Build history of the part. All positions in model axes, mm. Face numbers are marked on the shaded views. A direction names the side the tool comes from. Round coordinates to 2 decimals unless told otherwise and drop trailing zeros. Write each loop counter-clockwise with the first axis right and the second up, starting at its lowest first coordinate (ties: lowest second). Pieces come first, ordered by that corner, then holes. Notation, with made-up numbers: (49, 36) - (60, 36) arc R19 cw to (60, 46) - close; hole circle Ø6 at (37.5, 50). An arc over 180 degrees is marked (long way). Write each question's results on one line, items separated by ' | '.
from build123d import *

# Parameters (mm, degrees)
SKETCH1_W           = 32
SKETCH1_H           = 12
BOSS_EXTRUDE1_DEPTH = 2
SKETCH2_W           = 22
SKETCH2_H           = 12
BOSS_EXTRUDE2_DEPTH = 15
SKETCH3_W           = 22
SKETCH3_H           = 12
BOSS_EXTRUDE3_DEPTH = 4
BOSS_EXTRUDE4_DEPTH = 4
BOSS_EXTRUDE5_DEPTH = 4
SKETCH6_R           = 2.5
SKETCH6_R_2         = 0.75
BOSS_EXTRUDE6_DEPTH = 2
SKETCH7_R           = 1
SKETCH7_W           = 5
SKETCH7_H           = 1
CUT_EXTRUDE1_DEPTH  = 25.103941586
FILLET1_R           = 0.3
SKETCH8_W           = 1.18990991
SKETCH8_H           = 0.976336336
SKETCH8_H_2         = 0.976336337
BOSS_EXTRUDE7_DEPTH = 0.1


with BuildPart() as part:
    # Sketch1 → Boss-Extrude1 (new body)
    with BuildSketch(Plane(origin=(0, 0, 0), x_dir=(1, 0, 0), z_dir=(0, 1, 0))):
        Rectangle(SKETCH1_W, SKETCH1_H)
    extrude(amount=BOSS_EXTRUDE1_DEPTH)

    # Sketch2 → Boss-Extrude2 (add)
    with BuildSketch(Plane.XZ):
        Rectangle(SKETCH2_W, SKETCH2_H)
    extrude(amount=BOSS_EXTRUDE2_DEPTH)

    # Sketch3 → Boss-Extrude3 (add)
    with BuildSketch(Plane(origin=(0, 2, 0), x_dir=(1, 0, 0), z_dir=(0, 1, 0))):
        Rectangle(SKETCH3_W, SKETCH3_H)
    extrude(amount=BOSS_EXTRUDE3_DEPTH)

    # Sketch4 → Boss-Extrude4 (add)
    with BuildSketch(Plane(origin=(0, 6, 0), x_dir=(1, 0, 0), z_dir=(0, 1, 0))):
        with BuildLine():
            ThreePointArc((9.242640687, 4.242640687), (7.296100594, 5.543277195), (5, 6))
            ThreePointArc((5, 6), (0.757359313, 4.242640687), (-1, 0))
            ThreePointArc((-1, 0), (-0.543277195, -2.296100594), (0.757359313, -4.242640687))
            Line((0.757359313, -4.242640687), (9.242640687, 4.242640687))
        make_face()
        with BuildLine():
            ThreePointArc((11, 0), (10.543277195, 2.296100594), (9.242640687, 4.242640687))
            Line((9.242640687, 4.242640687), (0.757359313, -4.242640687))
            ThreePointArc((0.757359313, -4.242640687), (7.296100594, -5.543277195), (11, 0))
        make_face()
    extrude(amount=BOSS_EXTRUDE4_DEPTH)

    # Sketch5 → Boss-Extrude5 (add)
    with BuildSketch(Plane(origin=(0, 6, 0), x_dir=(1, 0, 0), z_dir=(0, 1, 0))):
        with BuildLine():
            ThreePointArc((-1, 0), (-0.862002062, 1.279426367), (-0.454356057, 2.5))
            Line((-0.454356057, 2.5), (-2, 2.5))
            ThreePointArc((-2, 2.5), (-4.5, 0), (-2, -2.5))
            Line((-2, -2.5), (-0.454356057, -2.5))
            ThreePointArc((-0.454356057, -2.5), (-0.862002062, -1.279426367), (-1, 0))
        make_face()
    extrude(amount=BOSS_EXTRUDE5_DEPTH)

    # Sketch6 → Boss-Extrude6 (add)
    with BuildSketch(Plane(origin=(0, 10, 0), x_dir=(1, 0, 0), z_dir=(0, 1, 0))):
        with Locations(Location((5, 0, 0), (0, 0, 270))):
            Circle(SKETCH6_R)
        with Locations(Location((5, 0, 0), (0, 0, 270))):
            Circle(SKETCH6_R_2, mode=Mode.SUBTRACT)
    extrude(amount=BOSS_EXTRUDE6_DEPTH)

    # Sketch7 → Cut-Extrude1 (cut, through all)
    with BuildSketch(Plane(origin=(0, 2, 0), x_dir=(1, 0, 0), z_dir=(0, 1, 0))):
        with Locations((14, 0)):
            Circle(SKETCH7_R)
        with Locations((-14, 0)):
            Circle(SKETCH7_R)
        with Locations((16, 0)):
            Rectangle(SKETCH7_W, SKETCH7_H)
        with Locations((-16, 0)):
            Rectangle(SKETCH7_W, SKETCH7_H)
    extrude(amount=-CUT_EXTRUDE1_DEPTH, mode=Mode.SUBTRACT)

    # Fillet1
    fillet1_edges = [part.edges().sort_by_distance(p)[0] for p in [
        (11, 4, -6),
        (11, -7.5, -6),
        (11, 4, 6),
        (11, -7.5, 6),
        (-11, 4, -6),
        (-11, 4, 6),
        (-11, -7.5, 6),
        (-11, -7.5, -6),
        (-16, 1, -6),
        (-16, 1, 6),
        (16, 1, -6),
        (16, 1, 6),
    ]]
    fillet(fillet1_edges, radius=FILLET1_R)

    # Sketch8 → Boss-Extrude7 (add)
    # profile 1 of 10: a face of its own
    with BuildSketch(Plane.XY.offset(6)):
        Polygon((-6.546228955, -2.789688189), (-7.217460186, -2.789688189), (-7.217460186, -1.581662663), (-7.868192168, -2.564673174), (-8.295339315, -2.564673174), (-8.926048774, -1.582616117), (-8.926048774, -2.775386387), (-9.597280006, -3.125303805), (-9.597280006, -0.837015516), (-8.876469195, -0.837015516), (-8.079858834, -1.98115966), (-7.268469946, -0.837015516), (-6.546228955, -0.837015516), align=None)
    # profile 2 of 10: a face of its own
    with BuildSketch(Plane.XY.offset(6)):
        Polygon((-5.569892618, -2.778246748), (-6.241123849, -3.125303805), (-6.241123849, -0.837015516), (-5.569892618, -0.837015516), align=None)
    # profile 3 of 10: a face of its own
    with BuildSketch(Plane.XY.offset(6)):
        Polygon((-2.923582558, -0.837015516), (-3.373135861, -1.325183685), (-4.624066792, -1.325183685), (-4.624066792, -2.301520021), (-2.99175448, -2.301520021), (-3.445121597, -2.789688189), (-4.84431454, -2.789688189), (-5.295298024, -2.344902153), (-5.295298024, -1.285138639), (-4.84431454, -0.837015516), align=None)
    # profile 4 of 10: a face of its own
    with BuildSketch(Plane.XY.offset(6)):
        Polygon((-0.2915743, -2.789688189), (-0.962805531, -2.789688189), (-0.962805531, -2.31772873), (-1.138717693, -2.148967468), (-2.152715441, -2.148967468), (-2.152715441, -2.770142393), (-2.823946672, -3.125303805), (-2.823946672, -0.837015516), (-0.762580306, -0.837015516), (-0.2915743, -1.45103954), (-0.63672445, -1.892488489), (-0.2915743, -2.219999751), align=None)
        Polygon((-0.981397873, -1.52397873), (-1.143008234, -1.325183685), (-2.152715441, -1.325183685), (-2.152715441, -1.6607993), (-1.096765741, -1.6607993), align=None, mode=Mode.SUBTRACT)
    # profile 5 of 10: a face of its own
    with BuildSketch(Plane.XY.offset(6)):
        Polygon((2.545903178, -2.332507258), (2.08824552, -2.789688189), (0.461653928, -2.789688189), (0.013530805, -2.342041793), (0.013530805, -1.285138639), (0.462130655, -0.837015516), (2.087768793, -0.837015516), (2.545903178, -1.294673174), align=None)
        with Locations((1.279716991, -1.813351853)):
            Rectangle(SKETCH8_W, SKETCH8_H, mode=Mode.SUBTRACT)
    # profile 6 of 10: a face of its own
    with BuildSketch(Plane.XY.offset(6)):
        Polygon((-1.064397577, -5.019272635), (-1.519194874, -5.623285398), (-3.801285715, -5.623285398), (-3.361266946, -5.13511723), (-1.916784964, -5.13511723), (-1.799033463, -5.025946809), (-1.91154097, -4.891033146), (-3.366987667, -4.891033146), (-3.801285715, -4.292741103), (-3.352685865, -3.670612725), (-1.064397577, -3.670612725), (-1.517764694, -4.158780893), (-2.964153583, -4.158780893), (-3.079044724, -4.29178765), (-2.963200129, -4.433375488), (-1.507753433, -4.433375488), align=None)
    # profile 7 of 10: a face of its own
    with BuildSketch(Plane.XY.offset(6)):
        Polygon((1.52994927, -3.670612725), (1.080395967, -4.158780893), (-0.170534964, -4.158780893), (-0.170534964, -4.433375488), (1.251540862, -4.433375488), (0.837265336, -4.891033146), (-0.170534964, -4.891033146), (-0.170534964, -5.13511723), (1.461777348, -5.13511723), (1.008410231, -5.623285398), (-0.841766195, -5.623285398), (-0.841766195, -3.670612725), align=None)
    # profile 8 of 10: a face of its own
    with BuildSketch(Plane.XY.offset(6)):
        Polygon((4.222978549, -5.623285398), (3.551747318, -5.623285398), (3.551747318, -5.151325938), (3.375835156, -4.982564677), (2.361837408, -4.982564677), (2.361837408, -5.603739602), (1.690606177, -5.958901013), (1.690606177, -3.670612725), (3.751972543, -3.670612725), (4.222978549, -4.284636749), (3.877828399, -4.726085698), (4.222978549, -5.053596959), align=None)
        Polygon((3.533154976, -4.357575938), (3.371544615, -4.158780893), (2.361837408, -4.158780893), (2.361837408, -4.494396509), (3.417787108, -4.494396509), align=None, mode=Mode.SUBTRACT)
    # profile 9 of 10: a face of its own
    with BuildSketch(Plane.XY.offset(6)):
        Polygon((7.226356928, -3.670612725), (6.175174495, -5.623285398), (5.574975546, -5.623285398), (4.528083654, -3.670612725), (5.194070892, -3.670612725), (5.874836657, -4.972553416), (6.555602423, -3.670612725), align=None)
    # profile 10 of 10: a face of its own
    with BuildSketch(Plane.XY.offset(6)):
        Polygon((9.989465036, -5.166104467), (9.531807378, -5.623285398), (7.905215787, -5.623285398), (7.457092663, -5.175639001), (7.457092663, -4.118735848), (7.905692513, -3.670612725), (9.531330651, -3.670612725), (9.989465036, -4.128270383), align=None)
        with Locations((8.72327885, -4.646949062)):
            Rectangle(SKETCH8_W, SKETCH8_H_2, mode=Mode.SUBTRACT)
    extrude(amount=BOSS_EXTRUDE7_DEPTH)


solid = part.part
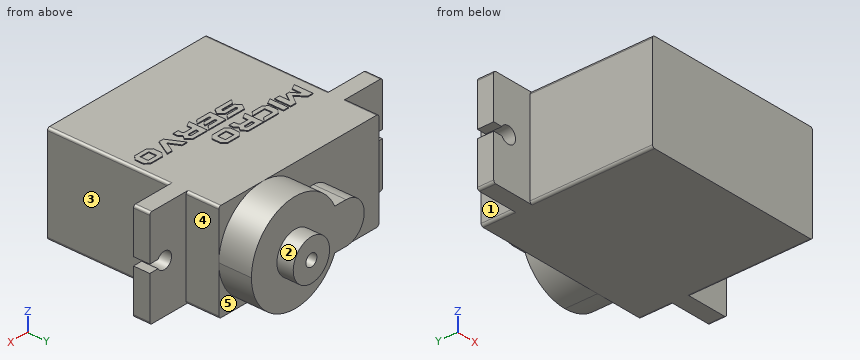
(1) Slice it at A-A, the plane x = -14. Write the cut outline in (y, z), and give its area (3 significant figures).
Worked answers:
outline: (0, -6) - (2, -6) - (2, -1) - (0, -1) - close; (0, 1) - (2, 1) - (2, 6) - (0, 6) - close | area: 20.0 mm2
(2) Tool access for the marked faces 1, 2, 3, 4 and 5: list every direction of +Z, -Z, +X, -X, +Y, -Y with a clear straight run to the whole face (end or side of a thin tool).
Worked answers:
face 1: +Z, -Z, -X, +Y | face 2: +Y | face 3: +Z, -Z, +X, -Y | face 4: +Z, -Z, +X, +Y | face 5: -Z, +X, +Y
(3) Slice it at B-B, the plane y = 9. Write the cut outline in (x, z), and give its area (3 significant figures).
Worked answers:
outline: (-2, -2.5) - (-0.45, -2.5) arc R6 ccw (long way) to (-0.45, 2.5) - (-2, 2.5) arc R2.5 ccw to start | area: 129 mm2
(4) Drill centre lines: probe 1 along Z at (x, y) = (14, 0.9); probe 2 along Y at (x, z) = (4, 3); probe 3 along Y at (x, z) = (-6, -2.25). Where is each one in solid material? Low to high. Write a range as [from, to].
Worked answers:
probe 1: z = [-6, -1], [1, 6] | probe 2: y = [-15, 10] | probe 3: y = [-15, 6]
(5) Flat gauge pins, fed straight in: pin 1 Ø2 at (x, y) = (-9, 1) entering from +Z; pin 2 Ø3.5 at (y, z) = (-8.5, -1) entering from -X; pin 3 Ø5 at (y, z) = (-6.5, 2) entering from +X. Where does each tip first touch, or does it go through?
Worked answers:
pin 1: stops at z = 6 | pin 2: stops at x = -11 | pin 3: stops at x = 11
